Read the model definition and answer for the solid it produces. Units are mm, in the model's axes. Face numbers are marked on the shaded views. A direction names the side the tool comes from. Coordinates: 2 decimals unless noted, no trailing zeros. Loops run counter-clockwise (first coordinate to the right, second up) from the corner with the lowest first, then second, coordinate; pieces in that order, holes last.
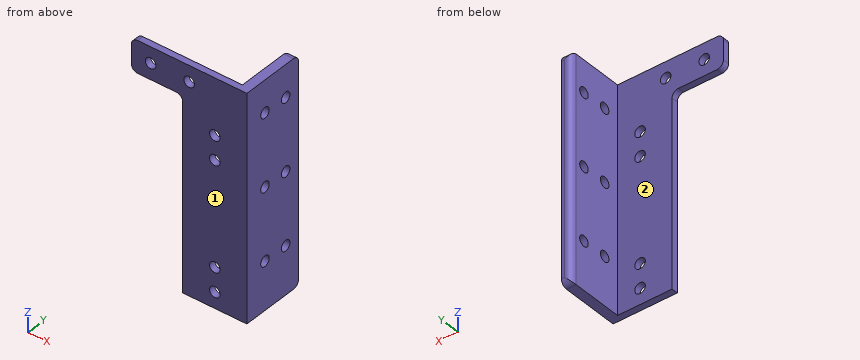
Autodesk Inventor part; units mm, degrees
ref_plane "YZ Plane" through (0, 0, 0) normal (1, 0, 0) x (0, 1, 0)
ref_plane "XZ Plane" through (0, 0, 0) normal (0, 1, 0) x (-1, 0, 0)
ref_plane "XY Plane" through (0, 0, 0) normal (0, 0, 1) x (1, 0, 0)
sketch "Sketch1" plane through (0, 0, 0) normal (0, 1, 0) x (-1, 0, 0)
  circle A0 centre (0, 0) radius 1.65
  circle A1 centre (-12, 0) radius 1.65
  circle A2 centre (-20, -12.5) radius 1.65
  circle A3 centre (-20, -52.5) radius 1.65
  line L0 (-10, -30) -> (-30, -30)
  line L1 (-30, -30) -> (-30, 5)
  line L2 (-30, 5) -> (-10, 5)
  line L3 (-10, 5) -> (-10, -30)
  line L4 (-10, -30) -> (-30, 5) construction
  line L5 (-30, -30) -> (-10, 5) construction
  line L6 (-30, -5) -> (6, -5)
  line L7 (6, -5) -> (6, 5)
  line L8 (6, 5) -> (-30, 5)
  line L9 (-30, 5) -> (-30, -5)
  line L10 (-30, -5) -> (6, 5) construction
  line L11 (6, -5) -> (-30, 5) construction
  line L12 (-10, -30) -> (-30, -30)
  line L13 (-30, -30) -> (-30, -65)
  line L14 (-30, -65) -> (-10, -65)
  line L15 (-10, -65) -> (-10, -30)
  line L16 (-30, 5) -> (-27, 5)
  line L17 (-27, 5) -> (-27, -65)
  line L18 (-27, -65) -> (-30, -65)
  line L19 (-30, -65) -> (-30, 5)
  circle A4 centre (-20, -20) radius 1.65
  circle A5 centre (-20, -60) radius 1.65
  point P0 (-10, -5)
  dimension "d0" = 3.3
  dimension "d1" = 3.3
  dimension "d2" = 12
  dimension "d3" = 3.3
  dimension "d4" = 12.5
  dimension "d5" = 20
  dimension "d6" = 3.3
  dimension "d7" = 40
  dimension "d8" = 20
  dimension "d9" = 35
  dimension "d25" = 3.3
  dimension "d26" = 20
  dimension "d27" = 3.3
  dimension "d28" = 40
extrude "Extrusion1" add sketch "Sketch1" along normal blind 2 contours L15 L14 L17 L0 | L0 L17 L6 L3 | L6 L17 L2 L3 | L3 L8 L7 L6
extrude "Extrusion2" add sketch "Sketch1" along normal blind 20 contours L17 L14 L13 L0 | L0 L1 L6 L17 | L6 L1 L2 L17
sketch "Sketch2" plane through (30, 0, 5) normal (1, 0, 0) x (0, 0, -1)
  circle A0 centre (10, 15) radius 1.65
  line L0 (0, 0) -> (0, 20)
  circle A1 centre (55, 15) radius 1.65
  line L1 (70, 0) -> (70, 20)
  circle A2 centre (32.5, 15) radius 1.65
  line L2 (0, 20) -> (70, 20)
  line L3 (0, 2) -> (0, 20)
  line L4 (0, 11) -> (70, 11)
  circle A3 centre (10, 7) radius 1.65
  circle A4 centre (55, 7) radius 1.65
  circle A5 centre (32.5, 7) radius 1.65
  point P0 (5, 0)
  point P1 (70, 10)
  dimension "d14" = 3.3
  dimension "d15" = 10
  dimension "d16" = 3.3
  dimension "d18" = 3.3
  dimension "d21" = 5
  dimension "d22" = 5
  dimension "d23" = 5
  dimension "d24" = 15
extrude "Extrusion3" cut sketch "Sketch2" against normal blind 20 contours A0 | A1 | A2 | A3 | A4 | A5
fillet "Fillet1" radius 2 6 edges at (-6, 1, -5) (10, 1, -5) (27, 20, -30) (28.5, 20, 5) (28.5, 20, -65) (-6, 1, 5)
properties part number "Holder Conveyor Kiri_3DPrint"
Item 1: Given pin 1 (1.5 mm diameter, centred on x = 19.5, z = -8, fed in from +Y); pin 2 (3 mm diameter, centred on x = 20, z = -12.5, fed in from -Y); pin 3 (5 mm diameter, centred on y = 11, z = -33, fed in from -X); pin 4 (1 mm diameter, centred on y = 1, z = -50, fed in from -X), each flat-ended and moving along its own axis, determine where each tip first touches the part or whether it passes through.
Numbers:
pin 1: stops at y = 2
pin 2: passes through
pin 3: stops at x = 27
pin 4: stops at x = 10
Item 2: A cutting plane is placed at D-D on x = 12. Determine the outline of the cut face in (y, z), then the cut area to 3 significant figures.
Numbers:
outline: (0, -65) - (2, -65) - (2, -1.65) - (0, -1.65) - close; (0, 1.65) - (2, 1.65) - (2, 5) - (0, 5) - close
area: 133 mm2
Item 3: Find the intervals of material crossed by line 1 along Z through (x, y) = (20, 0.9); line 2 along Y through (x, z) = (29, -50); line 3 along Y through (x, z) = (27.8, -50), in increasing order.
Numbers:
line 1: z = -65 to -61.65, -58.35 to -54.15, -50.85 to -21.65, -18.35 to -14.15, -10.85 to 5
line 2: y = 0 to 5.35, 8.65 to 13.35, 16.65 to 20
line 3: y = 0 to 5.35, 8.65 to 13.35, 16.65 to 19.6
Item 4: A cutting plane is placed at B-B on x = 0. Determine the outline of the cut face in (y, z).
Numbers:
outline: (0, -5) - (2, -5) - (2, -1.65) - (0, -1.65) - close; (0, 1.65) - (2, 1.65) - (2, 5) - (0, 5) - close
Item 5: A cutting plane is placed at C-C on z = -20. Determine the outline of the cut face in (x, y).
Numbers:
outline: (10, 0) - (18.35, 0) - (18.35, 2) - (10, 2) - close; (21.65, 0) - (30, 0) - (30, 20) - (29, 20) arc R2 ccw to (27, 18) - (27, 2) - (21.65, 2) - close
Item 6: Which of the six approach directions +Z, -Z, +X, -X, +Y, -Y give full straight-line access (tool end or side, diameter ignored) to the marked faces 1 and 2?
Numbers:
face 1: +Z, -Z, +X, -X, -Y
face 2: +Z, -Z, -X, +Y
Item 7: A cutting plane is placed at A-A on z = -27.5. Determine the outline of the cut face in (x, y).
Numbers:
outline: (10, 0) - (30, 0) - (30, 5.35) - (27, 5.35) - (27, 2) - (10, 2) - close; (27, 8.65) - (30, 8.65) - (30, 13.35) - (27, 13.35) - close; (27, 16.65) - (30, 16.65) - (30, 20) - (29, 20) arc R2 ccw to (27, 18) - close
